The listing builds one solid part. Answer for the finished solid, in the listing's coordinates (mm). A direction names the side the tool comes from. Give positions to 0.01 mm unless a question says otherwise; leave off trailing zeros. Order: outer loops, then holes, each group sorted by start corner. A loop starts at its lowest first (then second) coordinate and runs counter-clockwise, first axis right, second up. Notation, with made-up numbers: (27.5, -28.75) - (50.5, -28.75) arc R17 ccw to (50.5, -0.75) - close; hole circle Ø3 at (87, -4.75). An arc over 180 degrees is marked (long way). Answer as CSV lines item,"result". Start each with the question number.
1. Section A-A on z = 0 is taken. Give the vertices of the cut face in (x, y), and give its area (3 significant figures).
2. Which of the six approach directions +Z, -Z, +X, -X, +Y, -Y give full straight-line access (tool end or side, diameter ignored) to faces 3 (the flat face through (3, -7, 10)), 4 (the flat face through (-8.4, -3.1, 9.2)), 5 (the flat face through (-0.8, -1.5, 9.3))?
3. Consider line 1 along Z through (x, y) = (0.5, -10); line 2 along Z through (x, y) = (-0.5, -2); line 3 along X through (y, z) = (-14, -1). Determine where each line is inside the solid, lowest interval first. Write a range as [from, to].
4. Flat-ended cylindrical pins translate along their axes: pin 1 (4 mm diameter, centred on x = -6, y = -8.5, fed in from +Z); pin 2 (7 mm diameter, centred on x = 0, z = 0, fed in from +Y). Find the tip coordinate at first contact, or state that the pin passes through.
5. Determine the mould class of faces 1 (the flat face through (-9, -18, 10)), 2 (the flat face through (3, -16.4, 9.1)) for opening direction Y: +Y half, -Y half, draft (parallel to the pull), parting line (faces both ways), or undercut.
6. Section C-C on x = -8.25 is taken. Give the vertices of the cut face in (y, z).
7. Section B-B on y = -17.75 is taken. Give the vertices of the cut face in (x, z).
from build123d import *

# Parameters (mm, degrees)
F0_W     = 20
F0_H     = 20
F0_R     = 3
F1_DEPTH = 19.6
F2_SIZE  = 1
F4_DEPTH = 19.601
F6_DEPTH = 20.001


with BuildPart() as f1:
    # F0 (on Front) → F1 (new body)
    with BuildSketch(Plane.XZ):
        Rectangle(F0_W, F0_H)
        Circle(F0_R, mode=Mode.SUBTRACT)
    extrude(amount=F1_DEPTH)

    # F2
    f2_edges = [f1.edges().sort_by_distance(p)[0] for p in [
        (-3, -19.6, 0),
        (-3, 0, 0),
    ]]
    chamfer(f2_edges, length=F2_SIZE)

    # F3 (on face) → F4 (cut, through all)
    with BuildSketch(Plane.XZ.offset(19.6)):
        Polygon((-4.5, 10), (-7.5, 10), (-6, 8.5), align=None)
        Polygon((1.5, 10), (-1.5, 10), (0, 8.5), align=None)
        Polygon((7.5, 10), (4.5, 10), (6, 8.5), align=None)
    extrude(amount=-F4_DEPTH, mode=Mode.SUBTRACT)

    # F5 (on face) → F6 (cut, through all)
    with BuildSketch(Plane.YZ.offset(10)):
        Polygon((-14.3, 10), (-17.3, 10), (-15.8, 8.5), align=None)
        Polygon((-8.3, 10), (-11.3, 10), (-9.8, 8.5), align=None)
        Polygon((-2.3, 10), (-5.3, 10), (-3.8, 8.5), align=None)
    extrude(amount=-F6_DEPTH, mode=Mode.SUBTRACT)


solid = f1.part
Checks:
1,outline,"(-10, -19.6) - (-4, -19.6) - (-3, -18.6) - (-3, -1) - (-4, 0) - (-10, 0) - close; (3, -18.6) - (4, -19.6) - (10, -19.6) - (10, 0) - (4, 0) - (3, -1) - close"
1,area,"272 mm²"
2,face 3,"+Z, +X, -X, +Y, -Y"
2,face 4,"+Z, +X, -X"
2,face 5,"+Z, +Y, -Y"
3,line 1,"z = [-10, -2.96], [2.96, 8.7]"
3,line 2,"z = [-10, -2.96], [2.96, 9]"
3,line 3,"x = [-10, -2.83], [2.83, 10]"
4,pin 1,"stops at z = 10"
4,pin 2,"stops at y = -0.5"
5,face 1,"draft"
5,face 2,"undercut"
6,outline,"(-19.6, -10) - (0, -10) - (0, 10) - (-2.3, 10) - (-3.8, 8.5) - (-5.3, 10) - (-8.3, 10) - (-9.8, 8.5) - (-11.3, 10) - (-14.3, 10) - (-15.8, 8.5) - (-17.3, 10) - (-19.6, 10) - close"
7,outline,"(-10, -10) - (10, -10) - (10, 10) - (7.5, 10) - (6, 8.5) - (4.5, 10) - (1.5, 10) - (0, 8.5) - (-1.5, 10) - (-4.5, 10) - (-6, 8.5) - (-7.5, 10) - (-10, 10) - close; hole circle Ø6 at (0, 0)"
